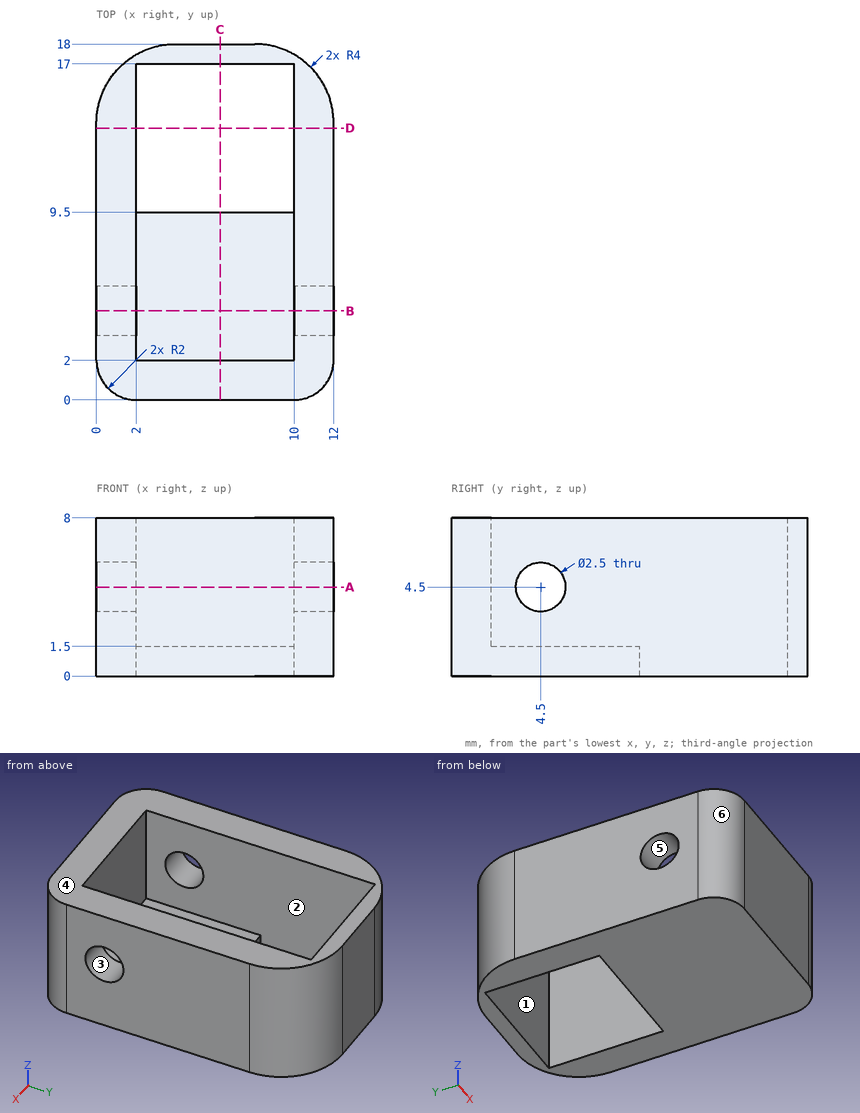
The drawing under review shows one solid part. Ordinate dimensions are in mm from its lowest x, y, z. A direction names the side the tool comes from. Coordinates: 2 decimals unless noted, no trailing zeros. Write each loop counter-clockwise with the first axis right and the second up, starting at its lowest first coordinate (ties: lowest second). Pieces come first, ordered by that corner, then holes. Notation, with made-up numbers: (48, 5) - (57, 5) arc R16 ccw to (57, 18) - close; hole circle Ø7 at (20.5, 14). An arc over 180 degrees is marked (long way). Answer in a Markdown table with one row per item. Add a question column.
Q1. For probe 1 along X at (y, z) = (11, 4.75); probe 2 along Y at (x, z) = (7.25, 4.75); probe 3 along Y at (x, z) = (11.1, 4.5), list the stretches that pass through material, from the lowest coordinate up.
Q2. Tool access review of the marked faces 1, 2 and 3: name each direction out of +Z, -Z, +X, -X, +Y, -Y from which nothing blocks a thin tool from reaching the whole face with its end or side.
Q3. We need section A-A, the plane z = 4.5. State the section outline as (x, y) points, and give its area (3 significant figures).
Q4. We need section C-C, the plane x = 6.25. State the section outline as (y, z) points.
Q5. We need section D-D, the plane y = 13.75. State the section outline as (x, z) points, and give its area (3 significant figures).
Q6. We need section B-B, the plane y = 4.5. State the section outline as (x, z) points.
Q7. Draft analysis for pull direction Z (two halves, no side actions). For the marked faces 4, 5 and 6, state which applies: +Z half, -Z half, draft (parallel to the pull), parting line (faces both ways), or undercut.
Q8. For P1, Ø2, axis at x = 6.5, y = 5.5, coming from the +Z side; P2, Ø3, axis at x = 1.5, z = 4.5, coming from the +Y side; P3, Ø2, axis at y = 4.5, z = 4.5, coming from the -X side, all flat-tipped, find the tip position at first contact; note any pin that passes through.
Answer list:
| question | item | result |
|---|---|---|
| 1 | probe 1 | x = 0 to 2, 10 to 12 |
| 1 | probe 2 | y = 0 to 2, 17 to 18 |
| 1 | probe 3 | y = 0.33 to 3.25, 5.75 to 16.53 |
| 2 | face 1 | +Z, -Z |
| 2 | face 2 | +Z |
| 2 | face 3 | +X, -X |
| 3 | outline | (0, 2) arc R2 ccw to (2, 0) - (10, 0) arc R2 ccw to (12, 2) - (12, 3.25) - (10, 3.25) - (10, 2) - (2, 2) - (2, 3.25) - (0, 3.25) - close; (0, 5.75) - (2, 5.75) - (2, 17) - (10, 17) - (10, 5.75) - (12, 5.75) - (12, 14) arc R4 ccw to (8, 18) - (4, 18) arc R4 ccw to (0, 14) - close |
| 3 | area | 77.4 mm2 |
| 4 | outline | (0, 0) - (9.5, 0) - (9.5, 1.5) - (2, 1.5) - (2, 8) - (0, 8) - close; (17, 0) - (18, 0) - (18, 8) - (17, 8) - close |
| 5 | outline | (0, 0) - (2, 0) - (2, 8) - (0, 8) - close; (10, 0) - (12, 0) - (12, 8) - (10, 8) - close |
| 5 | area | 32.0 mm2 |
| 6 | outline | (0, 0) - (12, 0) - (12, 3.25) - (10, 3.25) - (10, 1.5) - (2, 1.5) - (2, 3.25) - (0, 3.25) - close; (0, 5.75) - (2, 5.75) - (2, 8) - (0, 8) - close; (10, 5.75) - (12, 5.75) - (12, 8) - (10, 8) - close |
| 7 | face 4 | +Z half |
| 7 | face 5 | undercut |
| 7 | face 6 | draft |
| 8 | P1 | stops at z = 1.5 |
| 8 | P2 | stops at y = 17.87 |
| 8 | P3 | passes through |
